```python
from build123d import *

# Parameters (mm, degrees)
SKETCH1_R           = 3.2639
BOSS_EXTRUDE1_DEPTH = 4.7752


with BuildPart() as part:
    # Sketch1 (on Top Plane) → Boss-Extrude1 (new body)
    with BuildSketch(Plane(origin=(0, 0, 0), x_dir=(1, 0, 0), z_dir=(0, 1, 0))):
        Polygon((50.8, -47.3964), (50.8, 0), (0, 0), (0, -63.5), (22.907746615, -63.5), align=None)
        with Locations(Location((11.48588, -55.45328, 0), (0, 0, 90))):
            Circle(SKETCH1_R, mode=Mode.SUBTRACT)
        with Locations(Location((33.45942, -42.74312, 0), (0, 0, 90))):
            Circle(SKETCH1_R, mode=Mode.SUBTRACT)
        with Locations(Location((38.1, -12.7, 0), (0, 0, 90))):
            Circle(SKETCH1_R, mode=Mode.SUBTRACT)
        with Locations(Location((12.7, -12.7, 0), (0, 0, 90))):
            Circle(SKETCH1_R, mode=Mode.SUBTRACT)
    extrude(amount=-BOSS_EXTRUDE1_DEPTH)


solid = part.part
```
The model under review builds one solid part; all positions refer to its coordinate system, in mm. Give positions to 0.01 mm unless a question says otherwise; leave off trailing zeros. Write each loop counter-clockwise with the first axis right and the second up, starting at its lowest first coordinate (ties: lowest second). Pieces come first, ordered by that corner, then holes. Notation, with made-up numbers: M -21,61.25 L 32,61.25 A31 cw 32,90.25 Z; hole C 17,-23 d11. An arc over 180 degrees is marked long. Write item = value, one per line. Start each with the question number.
Q1. We need section C-C (z = 43.5). State the section outline as (x, y) points, plus the area to 3 significant figures.
Q2. For line 1 (X direction, y = -3, z = 12.7); line 2 (Z direction, x = 10.5, y = -3.95); line 3 (X direction, y = -1.3, z = 11), list the stretches that pass through material, from the lowest coordinate up.
Q3. We need section D-D (x = 12.7). State the section outline as (y, z) points, plus the area to 3 significant figures.
Q4. We need section B-B (x = 38.1). State the section outline as (y, z) points.
Q5. Mouldability with a two-part tool opening along X and no side actions: class faces 1 (the face through (41.286, -2.354, 13.408)), 2 (the face through (0, -2, 31)), 3 (the face through (36.66, -2.35, 55.56)), 4 (the face through (26, -2, 0)) as released by +X, released by -X, zero draft, split by the parting line, or undercut.
Q6. We need section A-A (z = 12.7). State the section outline as (x, y) points, plus the area to 3 significant figures.
Result set:
q1.outline = M 0,-4.78 L 30.28,-4.78 L 30.28,0 L 0,0 Z; M 36.63,-4.78 L 50.8,-4.78 L 50.8,0 L 36.63,0 Z
q1.area = 212 mm2
q2.line_1 = 0 to 9.44, 15.96 to 34.84, 41.36 to 50.8
q2.line_2 = 0 to 10.29, 15.11 to 52.34, 58.56 to 63.5
q2.line_3 = 0 to 9.91, 15.49 to 35.31, 40.89 to 50.8
q3.outline = M -4.78,0 L 0,0 L 0,9.44 L -4.78,9.44 Z; M -4.78,15.96 L 0,15.96 L 0,52.42 L -4.78,52.42 Z; M -4.78,58.48 L 0,58.48 L 0,63.5 L -4.78,63.5 Z
q3.area = 243 mm2
q4.outline = M -4.78,0 L 0,0 L 0,9.44 L -4.78,9.44 Z; M -4.78,15.96 L 0,15.96 L 0,54.73 L -4.78,54.73 Z
q5.face_1 = undercut
q5.face_2 = released by -X
q5.face_3 = released by +X
q5.face_4 = zero draft
q6.outline = M 0,-4.78 L 9.44,-4.78 L 9.44,0 L 0,0 Z; M 15.96,-4.78 L 34.84,-4.78 L 34.84,0 L 15.96,0 Z; M 41.36,-4.78 L 50.8,-4.78 L 50.8,0 L 41.36,0 Z
q6.area = 180 mm2
